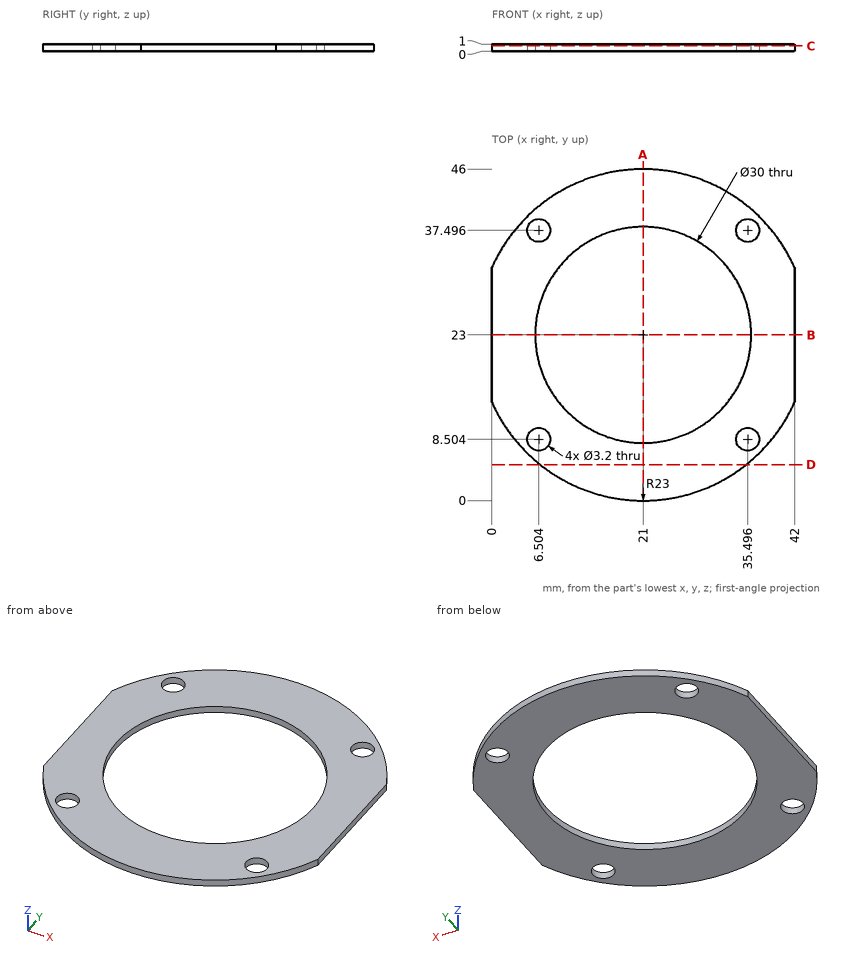
Geometry: see drawing. Coordinates: mm, zero at the bounding-box minimum. Round coordinates to 2 decimals unless told otherwise and drop trailing zeros. Write each loop counter-clockwise with the first axis right and the second up, starting at its lowest first coordinate (ties: lowest second). Pieces come first, ordered by that corner, then holes. Notation, with made-up numbers: M -22,-12 L 5,-12 A28 ccw 5,17 Z; hole C -28.5,64.5 d7. An arc over 180 degrees is marked long. Answer in a Markdown table with one row per item. Add a question column.
(1) Cut plane A-A, the plane x = 21. Return the cut outline in (y, z), then the cut area to 3 significant figures.
(2) Cut plane B-B, the plane y = 23. Return the cut outline in (x, z), then the cut area to 3 significant figures.
(3) Ray query, L1, parallel to Y at x = 21, z = 0.7; L2, parallel to X at y = 11, z = 0.5; L3, parallel to X at y = 32.5, z = 0.85 (1 decimal). Return the intervals inside material, ascending.
(4) Cut plane D-D, the plane y = 5. Return the cut outline in (x, z).
(5) Cut plane C-C, the plane z = 0.75. Return the cut outline in (x, y).
Established:
| question | item | result |
|---|---|---|
| 1 | outline | M 0,0 L 8,0 L 8,1 L 0,1 Z; M 38,0 L 46,0 L 46,1 L 38,1 Z |
| 1 | area | 16.0 mm² |
| 2 | outline | M 0,0 L 6,0 L 6,1 L 0,1 Z; M 36,0 L 42,0 L 42,1 L 36,1 Z |
| 2 | area | 12.0 mm² |
| 3 | L1 | 0 to 8, 38 to 46 |
| 3 | L2 | 1.38 to 12, 30 to 40.62 |
| 3 | L3 | 0.1 to 9.4, 32.6 to 41.9 |
| 4 | outline | M 6.68,0 L 35.32,0 L 35.32,1 L 6.68,1 Z |
| 5 | outline | M 0,13.62 A23 ccw 42,13.62 L 42,32.38 A23 ccw 0,32.38 Z; hole C 6.5,8.5 d3.2; hole C 6.5,37.5 d3.2; hole C 21,23 d30; hole C 35.5,8.5 d3.2; hole C 35.5,37.5 d3.2 |
